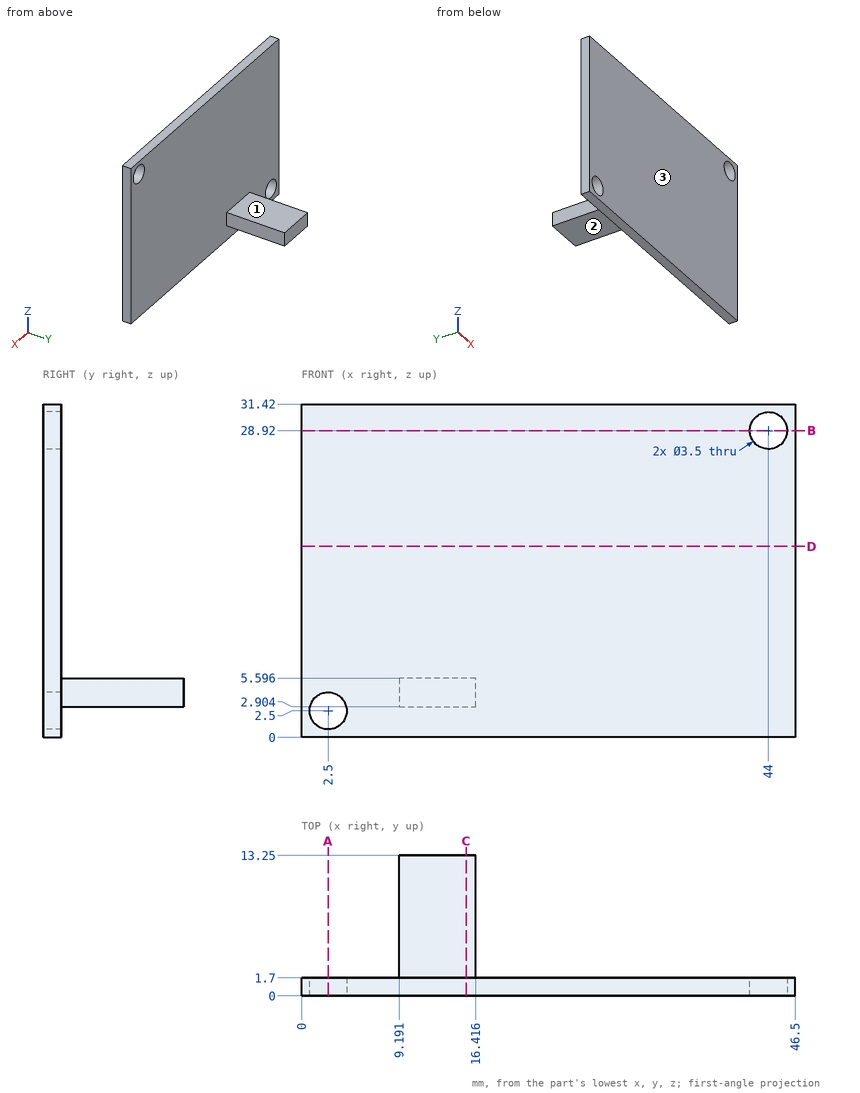
Verification items for this drawing (mm, ordinates from the low corner). A direction names the side the tool comes from. Round coordinates to 2 decimals unless told otherwise and drop trailing zeros. Write each loop counter-clockwise with the first axis right and the second up, starting at its lowest first coordinate (ties: lowest second). Pieces come first, ordered by that corner, then holes. Notation, with made-up numbers: (61, 46.5) - (90, 46.5) arc R26 cw to (90, 81.5) - close; hole circle Ø9 at (81, 19.25). An arc over 180 degrees is marked (long way). One line per item, written item: value.
1. Cross-section at C-C on x = 15.5. Record the boundary of the cut face in (y, z).
The answers:
outline: (0, 0) - (1.7, 0) - (1.7, 2.9) - (13.25, 2.9) - (13.25, 5.6) - (1.7, 5.6) - (1.7, 31.42) - (0, 31.42) - close
2. Cross-section at D-D on z = 18. Record the boundary of the cut face in (x, y).
The answers:
outline: (0, 0) - (46.5, 0) - (46.5, 1.7) - (0, 1.7) - close
3. Cross-section at B-B on z = 28.92. Record the boundary of the cut face in (x, y).
The answers:
outline: (0, 0) - (42.25, 0) - (42.25, 1.7) - (0, 1.7) - close; (45.75, 0) - (46.5, 0) - (46.5, 1.7) - (45.75, 1.7) - close
4. Cross-section at A-A on x = 2.5. Record the boundary of the cut face in (y, z).
The answers:
outline: (0, 0) - (1.7, 0) - (1.7, 0.75) - (0, 0.75) - close; (0, 4.25) - (1.7, 4.25) - (1.7, 31.42) - (0, 31.42) - close
5. Depth check by flat-ended pin: pin 1 Ø0.8 at (y, z) = (9, 4) entering from +X; pin 2 Ø3.5 at (x, y) = (12, 7.5) entering from +Z; pin 3 Ø4 at (x, z) = (2.5, 2.5) entering from +Y. Enter the tip coordinate at first touch or a pass-through.
The answers:
pin 1: stops at x = 16.42
pin 2: stops at z = 5.6
pin 3: stops at y = 1.7
6. Scan lines: L1, parallel to Z at x = 2.5, y = 0.6; L2, parallel to Z at x = 44, y = 1.3; L3, parallel to Y at x = 3, z = 10. Record each from-to range of solid material in increasing order.
The answers:
L1: z = 0 to 0.75, 4.25 to 31.42
L2: z = 0 to 27.17, 30.67 to 31.42
L3: y = 0 to 1.7
7. Set-up check for the marked faces 1, 2 and 3: record each of +Z, -Z, +X, -X, +Y, -Y from which the full face is reachable in a straight line by a thin tool's end or side.
The answers:
face 1: +Z, +X, -X, +Y
face 2: -Z, +X, -X, +Y
face 3: +Z, -Z, +X, -X, -Y
